Work out the finished part from the listing and answer in its coordinate system (mm). A direction names the side the tool comes from. Give positions to 0.01 mm unless a question says otherwise; leave off trailing zeros. Loops run counter-clockwise (first coordinate to the right, second up) from the corner with the lowest first, then second, coordinate; pieces in that order, holes last. Notation, with made-up numbers: M -22,38.25 L 4,38.25 A30 cw 4,74.25 Z; hole C 42.5,39 d4. An arc over 180 degrees is marked long. Answer as a JSON object with one key per item and string values. Group by question number.
Autodesk Inventor part; units mm, degrees
ref_plane "IDS_WORKPLANE{1}" through (-5.4001, 0, 0) normal (-1, 0, 0) x (0, 0, 1)
ref_plane "Work Plane3" through (1.25, 0, 0) normal (0, 0, 1) x (1, 0, 0)
ref_plane "YZ Plane" through (0, 0, 0) normal (1, 0, 0) x (0, 1, 0)
sketch "Sketch1" plane through (0, 0, 0) normal (0, 0, 1) x (1, 0, 0)
  line L0 (-1.3578, 4.8394) -> (-2.7, 1.1517)
  line L1 (-2.7, 1.1517) -> (-2.7, 0)
  line L2 (-2.7, 0) -> (25, 0)
  line L3 (25, 0) -> (25, 2.5)
  line L4 (25, 2.5) -> (0, 2.5)
  line L5 (0, 2.5) -> (0, 4.6)
  arc A0 (0, 4.6) -> (-1.3578, 4.8394) centre (-0.7, 4.6) ccw
  line L6 (-8.24, 0) -> (30.54, 0)
  line L7 (0, -1.0818) -> (0, 6.4909)
  dimension "d0" = 0.7
  dimension "d1" = 2.7
  dimension "d3" = 5
  dimension "d6" = 25
  dimension "d7" = 20
  dimension "d8" = 10.6
revolve "Body" add sketch "Sketch1" angle 360 about axis through (-2.7, 0, 0) along (1, 0, 0)
thread "Thread"
sketch "Sketch2" plane through (0, 0, 0) normal (1, 0, 0) x (0, 0, -1)
  circle A0 centre (0, 0) radius 4.6
  line L0 (0, 4.0415) -> (3.5, 2.0207)
  line L1 (3.5, 2.0207) -> (3.5, -2.0207)
  line L2 (3.5, -2.0207) -> (0, -4.0415)
  line L3 (0, -4.0415) -> (-3.5, -2.0207)
  line L4 (-3.5, -2.0207) -> (-3.5, 2.0207)
  line L5 (-3.5, 2.0207) -> (0, 4.0415)
  dimension "d14" = 7
extrude "Head" add sketch "Sketch2" against normal blind 5.4 contours L0 L1 L2 L3 L4 L5
fillet "Fillet1" radius 0.2 1 edges at (0, -2.5, 0)
ref_plane "IDS_WORKPLANE{1}" through (-5.4001, 0, 0) normal (-1, 0, 0) x (0, 0, 1)
sketch "Sketch3" plane through (-5.4001, 0, 0) normal (-1, 0, 0) x (0, 0, 1)
  circle A0 centre (0, 0) radius 3.1
  point P0 (0, 0)
  dimension "d18" = 6.2
extrude "Indent" cut sketch "Sketch3" against normal blind 1.401
sketch "Sketch4" plane through (0, 0, 0) normal (0, 0, 1) x (1, 0, 0)
  line L0 (-5.4, 3.5) -> (-5.4, 4.0415)
  line L1 (-5.4, 4.0415) -> (-5.0874, 4.0415)
  line L2 (-5.0874, 4.0415) -> (-5.4, 3.5)
  line L3 (-1.6482, 4.0415) -> (-5.4, 4.0415)
  line L4 (-5.4, 4.0415) -> (-5.4, 2.0207)
  line L5 (-6.1504, 0) -> (-0.8979, 0)
  dimension "d21" = 30
  dimension "d22" = 7
revolve "Chamfer1" cut sketch "Sketch4" angle 360 about axis through (-10, 0, 0) along (1, 0, 0)
ref_plane "Work Plane3" through (1.25, 0, 0) normal (0, 0, 1) x (1, 0, 0)
equation "\"d0\" = PHH"
equation "\"d1\" = 0.5 * KOH"
equation "\"d3\" = GD"
equation "\"d6\" = NLG"
equation "\"d7\" = KEWI"
equation "\"d8\" = LADI"
equation "\"d14\" = SW"
equation "\"d15\" = KOH"
equation "\"d18\" = KOD2"
equation "\"d21\" = ANG1"
equation "\"d22\" = SW"
equation "\"d9\" = GEL"
equation "\"d11\" = RR"
equation "\"NLG\" = 25"
equation "\"GD\" = NND"
equation "\"KOH\" = 5.4"
equation "\"GEL\" = 23.2"
equation "\"LADI\" = 10.6"
equation "\"SW\" = 7"
equation "\"PHH\" = 0.7"
equation "\"ANG1\" = 30deg"
equation "\"KEWI\" = 20deg"
equation "\"RR\" = 0.2"
equation "\"KOD2\" = 6.2"
equation "\"KOH2\" = 1.4"
equation "\"GUL\" = 0.61345 * PTC"
equation "\"SPD\" = 3.6"
equation "\"SD\" = 0"
equation "\"GD1\" = THREADDIA - 1.2269 * PTC"
equation "\"THREADDIA\" = 5"
equation "\"TOA\" = 30deg"
equation "\"BDM\" = NND"
equation "\"PTC\" = 0.8"
equation "\"NND\" = 5"
equation "\"BDM2\" = 4.36"
equation "\"GAL\" = 0.61345 * PTC"
equation "\"E0\" = 1.155 * SW"
properties part number "ANSI B 18.6.7 M / IFI 513 - M5x0,8 x 25, IHFHMSM" material "Steel, Mild"
Item 1: Given pin 1 Ø1.5 at (x, z) = (19, 0.5) entering from -Y; pin 2 Ø5 at (x, z) = (11, 2) entering from +Y; pin 3 Ø1.9 at (x, y) = (-3, 1) entering from +Z, each flat-ended and moving along its own axis, determine where each tip first touches the part or whether it passes through.
Item 2: For a pull along Z with two mould halves and no side action, classify faces 4 (the flat face through (-3, 0, -3.5)), 5 (the cylindrical face through (-4.71, -2.75, 1.43)), 6 (the conical face through (-5.324, 1.823, 3.141)) as pulls with the +Z half, pulls with the -Z half, needs draft (parallel to the pull), parting line crosses it, or undercut.
Item 3: Find the intervals of material crossed by probe 1 along X at (y, z) = (1.5, -3); probe 2 along X at (y, z) = (1.25, -2); probe 3 along Z at (x, y) = (-2, -1), in increasing order. Write a range as [from, to].
Item 4: A cutting plane is placed at A-A (x = -2.5). Determine the outline of the cut face in (y, z).
Item 5: A cutting plane is placed at B-B (x = 6.5). Determine the outline of the cut face in (y, z).
Item 6: A tool of negligible diameter and unlimited length cuts with its end or side. For faces 1 (the flat face through (0, 0, -3)), 2 (the flat face through (-3.5, -3, -1.8)), 3 (the flat face through (-3.5, 3, 1.8)), from which of +Z, -Z, +X, -X, +Y, -Y can it reach the whole face along a straight path? Write none if from no direction.
The answers:
{
 "1": {"pin 1": "stops at y = -2.5", "pin 2": "stops at y = 2.5", "pin 3": "stops at z = 3.5"},
 "2": {"face 4": "pulls with the -Z half", "face 5": "undercut", "face 6": "pulls with the +Z half"},
 "3": {"probe 1": "x = [-5.4, 0]", "probe 2": "x = [-4, 25]", "probe 3": "z = [-3.5, 3.5]"},
 "4": {"outline": "M -4.04,0 L -2.02,-3.5 L 2.02,-3.5 L 4.04,0 L 2.02,3.5 L -2.02,3.5 Z"},
 "5": {"outline": "C 0,0 d5"},
 "6": {"face 1": "+X", "face 2": "-Z, -X, -Y", "face 3": "+Z, -X, +Y"}
}
